```python
from build123d import *
from build123d.topology import SkipClean

# Parameters (mm, degrees)
SKETCH1_R            = 19.5
SKETCH1_R_2          = 18.5
BOSS_EXTRUDE1_DEPTH  = 15
SKETCH2_R            = 18.5
BOSS_EXTRUDE2_DEPTH  = 4
SKETCH3_R            = 18.5
CUT_EXTRUDE1_DEPTH   = 3
CUT_EXTRUDE2_DEPTH   = 3
CIRPATTERN1_COUNT    = 3
SKETCH8_R            = 4
BOSS_EXTRUDE28_DEPTH = 8
CUT_EXTRUDE3_DEPTH   = 8
SKETCH11_W           = 1
SKETCH11_H           = 15.24098
BOSS_EXTRUDE29_DEPTH = 8
CIRPATTERN5_COUNT    = 3
SKETCH12_W           = 1
SKETCH12_H           = 6.224425
BOSS_EXTRUDE30_DEPTH = 8
FILLET7_R            = 0.5
FILLET8_R            = 0.3


with BuildPart() as part:
    # Sketch1 → Boss-Extrude1 (new body)
    with BuildSketch(Plane(origin=(0, 0, 0), x_dir=(1, 0, 0), z_dir=(0, 1, 0))):
        with Locations(Location((0, 0, 0), (0, 0, 270))):
            Circle(SKETCH1_R)
        with Locations(Location((0, 0, 0), (0, 0, 270))):
            Circle(SKETCH1_R_2, mode=Mode.SUBTRACT)
    extrude(amount=BOSS_EXTRUDE1_DEPTH)

    # Sketch2 → Boss-Extrude2 (add)
    with BuildSketch(Plane(origin=(0, 0, 0), x_dir=(1, 0, 0), z_dir=(0, 1, 0))):
        with Locations(Location((0, 0, 0), (0, 0, 270))):
            Circle(SKETCH2_R)
    extrude(amount=BOSS_EXTRUDE2_DEPTH)

    # Sketch3 → Cut-Extrude1 (cut)
    with BuildSketch(Plane(origin=(0, 0, 0), x_dir=(-1, 0, 0), z_dir=(0, -1, 0))):
        with Locations(Location((0, 0, 0), (0, 0, 270))):
            Circle(SKETCH3_R)
    extrude(amount=-CUT_EXTRUDE1_DEPTH, mode=Mode.SUBTRACT)

    # Sketch6 → Cut-Extrude2 (cut)
    with BuildSketch(Plane(origin=(0, 3, 0), x_dir=(-1, 0, 0), z_dir=(0, -1, 0))):
        with BuildLine():
            ThreePointArc((-3.434212, 9.391815), (-1.743825, 9.84678), (0, 10))
            Line((0, 10), (0, 15.5))
            ThreePointArc((0, 15.5), (-1.76141, 15.399592), (-3.5, 15.099669))
            Line((-3.5, 15.099669), (-3.5, 9.391815))
            Line((-3.5, 9.391815), (-3.434212, 9.391815))
        make_face()
        with BuildLine():
            Line((0, 15.5), (0, 10))
            ThreePointArc((0, 10), (1.743825, 9.84678), (3.434212, 9.391815))
            Line((3.434212, 9.391815), (3.5, 9.391815))
            Line((3.5, 9.391815), (3.5, 15.099669))
            ThreePointArc((3.5, 15.099669), (1.76141, 15.399592), (0, 15.5))
        make_face()
    cut_extrude2 = extrude(amount=-CUT_EXTRUDE2_DEPTH, mode=Mode.SUBTRACT)

    # CirPattern1: Cut-Extrude2 ×3 about axis
    cirpattern1_axis = Axis((0, 0, 0), (0, 1, 0))
    for i in range(1, CIRPATTERN1_COUNT):
        add(cut_extrude2.rotate(cirpattern1_axis, i * 360 / CIRPATTERN1_COUNT), mode=Mode.SUBTRACT)

    # Sketch8 → Boss-Extrude28 (add)
    with BuildSketch(Plane.XZ.offset(-3)):
        with Locations(Location((0, 0, 0), (0, 0, 270))):
            Circle(SKETCH8_R)
        with BuildLine():
            Line((-2, -2.236068), (-2, 2.236068))
            ThreePointArc((-2, 2.236068), (3, 0), (-2, -2.236068))
        make_face(mode=Mode.SUBTRACT)
    extrude(amount=-BOSS_EXTRUDE28_DEPTH)

    # Sketch8<3> → Cut-Extrude3 (cut)
    with SkipClean():  # the faces are left unmerged after this step: merging them gives an invalid solid
        with BuildSketch(Plane.XZ.offset(-3)):
            with BuildLine():
                ThreePointArc((3, 0), (1.224745, 2.738613), (-2, 2.236068))
                Line((-2, 2.236068), (-2, -2.236068))
                ThreePointArc((-2, -2.236068), (1.224745, -2.738613), (3, 0))
            make_face()
        extrude(amount=-CUT_EXTRUDE3_DEPTH, mode=Mode.SUBTRACT)

    # Sketch11 → Boss-Extrude29 (add)
    with SkipClean():  # the faces are left unmerged after this step: merging them gives an invalid solid
        with BuildSketch(Plane(origin=(0, 11, 0), x_dir=(1, 0, 0), z_dir=(0, 1, 0))):
            with Locations((0, -11.25)):
                Rectangle(SKETCH11_W, SKETCH11_H)
        boss_extrude29 = extrude(amount=-BOSS_EXTRUDE29_DEPTH)

    # CirPattern5: Boss-Extrude29 ×3 about axis
    with SkipClean():  # the faces are left unmerged after this step: merging them gives an invalid solid
        cirpattern5_axis = Axis((0, 0, 0), (0, 1, 0))
        for i in range(1, CIRPATTERN5_COUNT):
            add(boss_extrude29.rotate(cirpattern5_axis, i * 360 / CIRPATTERN5_COUNT))

    # Sketch12 → Boss-Extrude30 (add)
    with SkipClean():  # the faces are left unmerged after this step: merging them gives an invalid solid
        with BuildSketch(Plane.XZ):
            with Locations((0, 15.612213)):
                Rectangle(SKETCH12_W, SKETCH12_H)
        extrude(amount=-BOSS_EXTRUDE30_DEPTH)

    # Fillet7
    fillet7_edges = [part.edges().sort_by_distance(p)[0] for p in [
        (-0.5, 1.5, 12.5),
        (0.5, 1.5, 12.5),
    ]]
    fillet(fillet7_edges, radius=FILLET7_R - 0.0001)  # a hair under: the kernel refuses the full size

    # Fillet8
    fillet8_edges = [part.edges().sort_by_distance(p)[0] for p in [
        (0, 0, -19.5),
        (0, 0, -18.5),
        (-0.5, 0, 15.746571),
        (0.5, 0, 15.746571),
        (0.353583, 0, 12.646417),
        (-0.353583, 0, 12.646417),
    ]]
    fillet(fillet8_edges, radius=FILLET8_R)


solid = part.part
```
Can you work these out from the model? Positions are in its coordinate system, mm. A direction names the side the tool comes from. Coordinates: 2 decimals unless noted, no trailing zeros. Loops run counter-clockwise (first coordinate to the right, second up) from the corner with the lowest first, then second, coordinate; pieces in that order, holes last.
Item 1: Suppose I cut it at D-D (y = 12.75). Please give me the cut outline in (x, z).
Answers below:
outline: circle Ø39 at (0, 0); hole circle Ø37 at (0, 0)
Item 2: If we mould it in two halves opening along X, with no side actions, what happens to faces 4 (the face through (-8.821, 3.493, 9.134)), 5 (the face through (-7.13, 15, 17.24))? For each: released by +X, released by -X, zero draft, split by the parting line, or undercut.
Answers below:
face 4: undercut
face 5: zero draft
Item 3: Suppose I cut it at A-A (y = 9.75). Please give me the cut outline in (x, z).
Answers below:
outline: circle Ø39 at (0, 0); hole (-16.27, -8.81) - (-3.69, -1.55) arc R4 cw to (-0.5, 3.97) - (-0.5, 18.49) arc R18.5 ccw to start; hole (-15.77, -9.68) arc R18.5 ccw to (15.77, -9.68) - (3.19, -2.42) arc R4 cw to (-3.19, -2.42) - close; hole (-2, -2.24) arc R3 ccw (long way) to (-2, 2.24) - close; hole (0.5, 3.97) arc R4 cw to (3.69, -1.55) - (16.27, -8.81) arc R18.5 ccw to (0.5, 18.49) - close
Item 4: I'm going to push flat-ended pins straight in: pin 1 (1.1 mm diameter, centred on y = 3.5, z = -11.5, fed in from +X); pin 2 (4 mm diameter, centred on x = 15, y = 9.5, fed in from +Z); pin 3 (3 mm diameter, centred on x = -11, y = 13, fed in from -Z). Where does each tip first touch, or does it pass through?
Answers below:
pin 1: stops at x = 16.14
pin 2: stops at z = 14.53
pin 3: stops at z = -17.03
Item 5: Which directions (+Z, -Z, +X, -X, +Y, -Y) give clear straight access to the entire face, cutting with the end or side of a thin tool? Please do faces 1 (the face through (9.564, 7.549, -6.099)), 2 (the face through (-0.5, 2, 16)), 3 (the face through (3.5, 3.5, -12.3)).
Answers below:
face 1: +Y
face 2: -Y
face 3: +Y, -Y
Item 6: Suppose I cut it at C-C (x = 1.5). State how many separate pieces and enclosed holes the cut face has, then the cut area to 3 significant figures.
Answers below:
separate pieces: 3
enclosed holes: 0
area: 71.7 mm2
Item 7: Please list where these lines run through material, in increasing order: L1, parallel to X at y = 9, z = 0; L2, parallel to Z at x = 4.5, y = 8.25; L3, parallel to X at y = 1.5, z = 0.
Answers below:
L1: x = -19.5 to -18.5, -4 to -2, 3 to 4, 18.5 to 19.5
L2: z = -18.97 to -17.94, -3.18 to -2.02, 17.94 to 18.97
L3: x = -19.5 to -18.5, 18.5 to 19.5
